Read the model definition and answer for the solid it produces. Units are mm, in the model's axes. Face numbers are marked on the shaded views. A direction names the side the tool comes from. Coordinates: 2 decimals unless noted, no trailing zeros. Write each loop counter-clockwise with the first axis right and the second up, starting at its lowest first coordinate (ties: lowest second). Pieces come first, ordered by that corner, then holes. Notation, with made-up numbers: (21, 4) -> (72, 4) arc R34 ccw to (72, 39) -> close; hole circle Ø5 at (-20, 50). An arc over 180 degrees is marked (long way). One line per item, written item: value. Start each with the question number.
1. Find section D-D, the plane z = 10.5. Write down the section's boundary in (x, y).
2. Given P1, Ø1.8, axis at x = -22, z = 14.5, coming from the -Y side; P2, Ø11, axis at y = -7, z = 3.5, coming from the +X side; P3, Ø1.5, axis at x = 3, y = 1, coming from the +Z side, each flat-ended and moving along its own axis, determine where each tip first touches the part or whether it passes through.
3. For the marked faces 5, 6 and 7, determine the directions among +Z, -Z, +X, -X, +Y, -Y from which every point of the face is accessible in a straight line to the end or side of a thin tool.
4. For a pull along Z with two mould halves and no side action, classify the marked faces 1, 2, 3 and 4 as pulls with the +Z half, pulls with the -Z half, needs draft (parallel to the pull), parting line crosses it, or undercut.
5. Find section C-C, the plane x = 1.5. Write down the section's boundary in (y, z).
6. Find section B-B, the plane z = 0. Write down the section's boundary in (x, y).
7. Consider line 1 along Y through (x, z) = (23, 0); line 2 along X through (y, z) = (4, 15); line 3 along Z through (x, y) = (23, -7). Determine where each line is inside the solid, lowest interval first.
8. Find section A-A, the plane y = 0. Write down the section's boundary in (x, z), and give its area (3 significant figures).
```python
from build123d import *

# Parameters (mm, degrees)
SKETCH_1_R          = 18.3
EXTRUDE_1_DEPTH     = 26.4
SKETCH_4_R          = 16.5
EXTRUDE_2_DEPTH     = 19
SKETCH_5_R          = 15.25
EXTRUDE_3_DEPTH     = 1
SKETCH_6_R          = 6.9
EXTRUDE_4_DEPTH     = 6
SKETCH_7_W          = 7
SKETCH_7_H          = 12
EXTRUDE_5_DEPTH     = 6
SKETCH_3_R          = 1.5
CUT_EXTRUDE_7_DEPTH = 4
SKETCH_18_R         = 6
EXTRUDE_7_DEPTH     = 6
SKETCH_19_R         = 3
EXTRUDE_9_DEPTH     = 2
EXTRUDE_10_DEPTH    = 9


with BuildPart() as part:
    # 草图1 → 凸台-拉伸1 (new body)
    with BuildSketch(Plane(origin=(0, 0, 0), x_dir=(0, 0, -1), z_dir=(1, 0, 0))):
        Circle(SKETCH_1_R)
    extrude(amount=EXTRUDE_1_DEPTH)

    # 草图4 → 凸台-拉伸2 (add)
    with BuildSketch(Plane.ZY):
        Circle(SKETCH_4_R)
    extrude(amount=EXTRUDE_2_DEPTH)

    # 草图5 → 凸台-拉伸3 (add)
    with BuildSketch(Plane.ZY.offset(19)):
        Circle(SKETCH_5_R)
    extrude(amount=EXTRUDE_3_DEPTH)

    # 草图6 → 凸台-拉伸4 (add)
    with BuildSketch(Plane.ZY.offset(20)):
        Circle(SKETCH_6_R)
    extrude(amount=EXTRUDE_4_DEPTH)

    # 草图7 → 凸台-拉伸5 (add)
    with BuildSketch(Plane.ZY.offset(20)):
        with Locations((13, 0)):
            Rectangle(SKETCH_7_W, SKETCH_7_H)
    extrude(amount=EXTRUDE_5_DEPTH)

    # 草图3 → 切除-拉伸7 (cut)
    with BuildSketch(Plane(origin=(26.4, 0, 0), x_dir=(0, 0, -1), z_dir=(1, 0, 0))):
        with Locations((-13.423393759, 7.75)):
            Circle(SKETCH_3_R)
        with Locations((-13.423393759, -7.75)):
            Circle(SKETCH_3_R)
        with Locations((0, -15.5)):
            Circle(SKETCH_3_R)
        with Locations((13.423393759, -7.75)):
            Circle(SKETCH_3_R)
        with Locations((13.423393759, 7.75)):
            Circle(SKETCH_3_R)
        with Locations((0, 15.5)):
            Circle(SKETCH_3_R)
    extrude(amount=-CUT_EXTRUDE_7_DEPTH, mode=Mode.SUBTRACT)

    # 草图18 → 凸台-拉伸7 (add)
    with BuildSketch(Plane(origin=(26.4, 0, 0), x_dir=(0, 0, -1), z_dir=(1, 0, 0))):
        with Locations((7.396149949, 0)):
            Circle(SKETCH_18_R)
    extrude(amount=EXTRUDE_7_DEPTH)

    # 草图19 → 凸台-拉伸9 (add)
    with BuildSketch(Plane(origin=(32.4, 0, 0), x_dir=(0, 0, -1), z_dir=(1, 0, 0))):
        with Locations((7.396149949, 0)):
            Circle(SKETCH_19_R)
    extrude(amount=EXTRUDE_9_DEPTH)

    # 草图23 → 凸台-拉伸10 (add)
    with BuildSketch(Plane(origin=(34.4, 0, 0), x_dir=(0, 0, -1), z_dir=(1, 0, 0))):
        with BuildLine():
            Line((5.737938338, 2.500066849), (9.054361561, 2.500066849))
            ThreePointArc((9.054361561, 2.500066849), (7.396149949, -3), (5.737938338, 2.500066849))
        make_face()
    extrude(amount=EXTRUDE_10_DEPTH)


solid = part.part
```
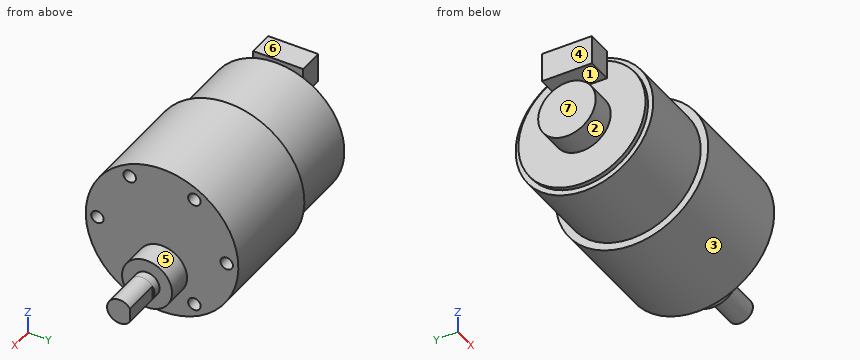
Answer block:
1. outline: (-26, -6) -> (-20, -6) -> (-20, -11.06) -> (-19, -11.06) -> (-19, -12.73) -> (0, -12.73) -> (0, -14.99) -> (26.4, -14.99) -> (26.4, 14.99) -> (0, 14.99) -> (0, 12.73) -> (-19, 12.73) -> (-19, 11.06) -> (-20, 11.06) -> (-20, 6) -> (-26, 6) -> close
2. P1: stops at y = -6
2. P2: stops at x = 26.4
2. P3: stops at z = 18.3
3. face 5: +X
3. face 6: +Z, -X, +Y, -Y
3. face 7: +Z, -Z, -X, +Y, -Y
4. face 1: undercut
4. face 2: undercut
4. face 3: parting line crosses it
4. face 4: needs draft
5. outline: circle Ø36.6 at (0, 0)
6. outline: (-26, -6.9) -> (-20, -6.9) -> (-20, -15.25) -> (-19, -15.25) -> (-19, -16.5) -> (0, -16.5) -> (0, -18.3) -> (26.4, -18.3) -> (26.4, -17) -> (22.4, -17) -> (22.4, -14) -> (26.4, -14) -> (26.4, 14) -> (22.4, 14) -> (22.4, 17) -> (26.4, 17) -> (26.4, 18.3) -> (0, 18.3) -> (0, 16.5) -> (-19, 16.5) -> (-19, 15.25) -> (-20, 15.25) -> (-20, 6.9) -> (-26, 6.9) -> close
7. line 1: y = -18.3 to -17, -14 to 14, 17 to 18.3
7. line 2: x = -26 to -20, -19 to 26.4
7. line 3: z = -16.91 to -14.72, -12.12 to 12.12, 14.72 to 16.91
8. outline: (-26, -6.9) -> (-20, -6.9) -> (-20, -15.25) -> (-19, -15.25) -> (-19, -16.5) -> (0, -16.5) -> (0, -18.3) -> (26.4, -18.3) -> (26.4, -13.4) -> (32.4, -13.4) -> (32.4, -10.4) -> (43.4, -10.4) -> (43.4, -4.4) -> (32.4, -4.4) -> (32.4, -1.4) -> (26.4, -1.4) -> (26.4, 18.3) -> (0, 18.3) -> (0, 16.5) -> (-19, 16.5) -> (-19, 15.25) -> (-20, 15.25) -> (-20, 16.5) -> (-26, 16.5) -> (-26, 9.5) -> (-20, 9.5) -> (-20, 6.9) -> (-26, 6.9) -> close
8. area: 1,890 mm2
